```python
from build123d import *

# Parameters (mm, degrees)
BOSS_EXTRUDE1_DEPTH      = 2
BOSS_EXTRUDE2_DEPTH      = 19
BOSS_EXTRUDE2_DEPTH_BACK = 19
SKETCH3_W                = 100
SKETCH3_H                = 63
BOSS_EXTRUDE3_START      = -44
SKETCH6_W                = 90
SKETCH6_H                = 37
BOSS_EXTRUDE3_DEPTH      = 88


with BuildPart() as part:
    # Sketch2 → Boss-Extrude1 (new body)
    with BuildSketch(Plane(origin=(0, 0, 0), x_dir=(1, 0, 0), z_dir=(0, 1, 0))):
        Polygon((-27, 0), (27, 0), (27, 54), (80, 54), (80, 122), (66, 122), (66, 172), (55, 172), (55, 247), (44, 247), (44, 328), (-44, 328), (-44, 247), (-55, 247), (-55, 172), (-66, 172), (-66, 122), (-80, 122), (-80, 54), (-27, 54), align=None)
    extrude(amount=BOSS_EXTRUDE1_DEPTH)

    # Sketch3 → Boss-Extrude2 (add, two sides: drawn at the far end of the back side and taken through both)
    with BuildSketch(Plane(origin=(0, 0, 0), x_dir=(0, 0, -1), z_dir=(1, 0, 0)).offset(-BOSS_EXTRUDE2_DEPTH_BACK)):
        with Locations((50, 33.5)):
            Rectangle(SKETCH3_W, SKETCH3_H)
    extrude(amount=BOSS_EXTRUDE2_DEPTH + BOSS_EXTRUDE2_DEPTH_BACK)

    # Sketch6 → Boss-Extrude3 (add)
    with BuildSketch(Plane(origin=(0, 0, 0), x_dir=(0, 0, -1), z_dir=(1, 0, 0)).offset(BOSS_EXTRUDE3_START)):
        with Locations((283, 20.5)):
            Rectangle(SKETCH6_W, SKETCH6_H)
    extrude(amount=BOSS_EXTRUDE3_DEPTH)


solid = part.part
```
The model under review builds one solid part; all positions refer to its coordinate system, in mm. A direction names the side the tool comes from. Round coordinates to 2 decimals unless told otherwise and drop trailing zeros. Order: outer loops, then holes, each group sorted by start corner. A loop starts at its lowest first (then second) coordinate and runs counter-clockwise, first axis right, second up. Notation, with made-up numbers: (85, 57) -> (129, 57) arc R25 ccw to (129, 75) -> close; hole circle Ø9 at (34, 0). An arc over 180 degrees is marked (long way). One line per item, written item: value. Start each with the question number.
Q1. Take a section at A-A (y = 27.5). Write out the cut boundary in (x, z), and give its area (3 significant figures).
Q2. Clearance check with flat-ended pins moving along their axes: pin 1 Ø0.6 at (x, y) = (-69.5, 1) entering from -Z; pin 2 Ø1 at (x, y) = (-46, 1.5) entering from +Z; pin 3 Ø3 at (x, z) = (23, -207) entering from +Y. State where each tip first meets the part, or that it passes through.
Q3. Take a section at B-B (z = -91). Write out the cut boundary in (x, y).
Q4. Take a section at D-D (y = 54). Write out the cut boundary in (x, z).
Q5. Machinability: for faces 1 (the face through (19, 34, -49)), 2 (the face through (-1, 20, -238)), 3 (the face through (-19, 34, -49)), 4 (the face through (-1, 39, -282)), which of the approach directions +Z, -Z, +X, -X, +Y, -Y give a long, thin tool a straight path to every point of the face, cutting with its end or side? Answer none if there is none.
Q6. Wall thickness on line 1 (X direction, y = 32, z = -85); line 2 (Z direction, x = -20.5, y = 20); line 3 (Y direction, x = 20, z = -261): over which ranges is each line inside the solid? List them lowest first.
Q7. Take a section at C-C (x = 11). Write out the cut boundary in (y, z).
Reported:
1. outline: (-44, -328) -> (44, -328) -> (44, -238) -> (-44, -238) -> close; (-19, -100) -> (19, -100) -> (19, 0) -> (-19, 0) -> close
1. area: 11,700 mm2
2. pin 1: stops at z = -122
2. pin 2: stops at z = -54
2. pin 3: stops at y = 2
3. outline: (-80, 0) -> (80, 0) -> (80, 2) -> (19, 2) -> (19, 65) -> (-19, 65) -> (-19, 2) -> (-80, 2) -> close
4. outline: (-19, -100) -> (19, -100) -> (19, 0) -> (-19, 0) -> close
5. face 1: +Z, +X, +Y
5. face 2: +X, -X, +Y
5. face 3: +Z, -X, +Y
5. face 4: -Z, +X, -X, +Y
6. line 1: x = -19 to 19
6. line 2: z = -328 to -238
6. line 3: y = 0 to 39
7. outline: (0, -328) -> (39, -328) -> (39, -238) -> (2, -238) -> (2, -100) -> (65, -100) -> (65, 0) -> (0, 0) -> close
